```python
from build123d import *

# Parameters (mm, degrees)
F0_R     = 18.034415
F1_DEPTH = 14.986
F2_R     = 5.08


with BuildPart() as f1:
    # F0 (on Top) → F1 (new body)
    with BuildSketch(Plane.XY):
        Circle(F0_R)
    extrude(amount=F1_DEPTH)

    # F2
    f2_edges = [f1.edges().sort_by_distance(p)[0] for p in [
        (18.034415, 0, 7.493),
        (-18.034415, 0, 0),
        (-18.034415, 0, 14.986),
    ]]
    fillet(f2_edges, radius=F2_R)

    # F3 (on Right) → F4 (revolve, cut)
    with BuildSketch(Plane.YZ):
        with BuildLine():
            Line((-41.504344, 55.164188), (41.504344, 55.164188))
            ThreePointArc((41.504344, 55.164188), (0, 96.668532), (-41.504344, 55.164188))
        make_face()
    revolve(axis=Axis((0, 0.253545, 55.164188), (0, -1, 0)), mode=Mode.SUBTRACT)

    # F5 (on Front) → F6 (revolve, cut)
    with BuildSketch(Plane.XZ):
        with BuildLine():
            ThreePointArc((-38.461781, -37.017379), (0, -75.47916), (38.461781, -37.017379))
            Line((38.461781, -37.017379), (-38.461781, -37.017379))
        make_face()
    revolve(axis=Axis((1.748852, 0, -37.017379), (-1, 0, 0)), mode=Mode.SUBTRACT)


solid = f1.part
```
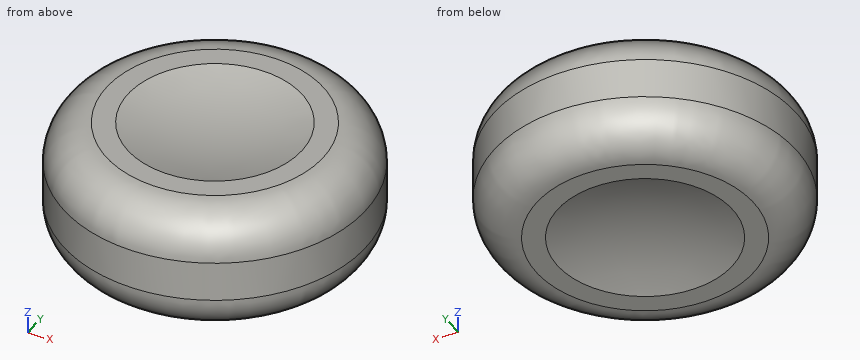
Build history of the part. All positions in model axes, mm. Give positions to 0.01 mm unless a question says otherwise; leave off trailing zeros. Order: outer loops, then holes, each group sorted by start corner. A loop starts at its lowest first (then second) coordinate and runs counter-clockwise, first axis right, second up. Notation, with made-up numbers: M -34,-2 L -23,-2 A15 ccw -23,11 Z; hole C -2,34 d1. An arc over 180 degrees is marked long. Write item = value, one per line. Start each with the question number.
(1) Slice it at A-A on y = 0. Write the cut outline in (x, z).
(2) Pin check, flat tips, straight feed: pin 1 Ø8 at (y, z) = (-11, 12) entering from -X; pin 2 Ø1 at (x, y) = (-5.5, -5) entering from +Z; pin 3 Ø1 at (x, z) = (-11, 10.5) entering from +Y. Stop position of each tip, or through.
(3) Probe L1, parallel to X at y = 13, z = 11.25; L2, parallel to X at y = 15, z = 3.25; L3, parallel to Z at x = -5, y = 1. List the from-to ranges inside material, lowest first. Write a range as [from, to].
(4) Slice it at C-C on z = 7. Write the cut outline in (x, y).
Responses:
q1.outline = M -18.03,5.08 A5.08 ccw -12.95,0 L -10.44,0 A38.46 cw 10.44,0 L 12.95,0 A5.08 ccw 18.03,5.08 L 18.03,9.91 A5.08 ccw 12.95,14.99 L 10.41,14.99 A41.5 cw -10.41,14.99 L -12.95,14.99 A5.08 ccw -18.03,9.91 Z
q2.pin_1 = -16.46
q2.pin_2 = 14.43
q2.pin_3 = 14.63
q3.L1 = [-12.24, 12.24]
q3.L2 = [-9.38, 9.38]
q3.L3 = [1.1, 13.97]
q4.outline = C 0,0 d36.07
